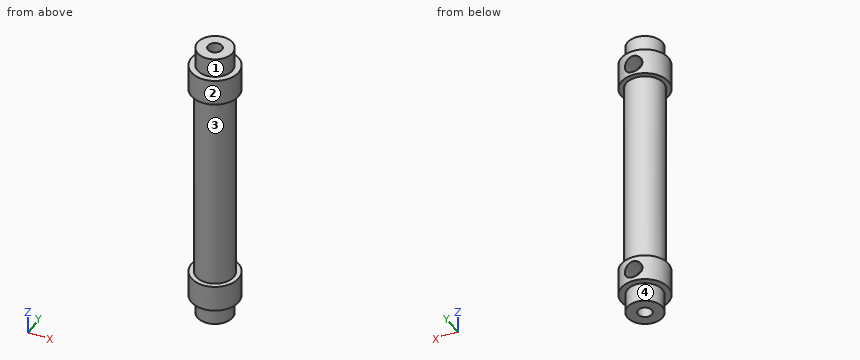
from build123d import *

# Parameters (mm, degrees)
SKETCH_1_R          = 10.75
SKETCH_1_R_2        = 9
EXTRUDE_1_DEPTH     = 115
SKETCH_2_R          = 13.5
EXTRUDE_2_DEPTH     = 15
SKETCH_3_R          = 10
EXTRUDE_3_DEPTH     = 11
SKETCH_4_R          = 4
CUT_EXTRUDE_4_DEPTH = 143.286682441
SKETCH_5_R          = 5
CUT_EXTRUDE_5_DEPTH = 15


with BuildPart() as part:
    # 草图1 → 拉伸1 (new body)
    with BuildSketch(Plane.XY):
        Circle(SKETCH_1_R)
        Circle(SKETCH_1_R_2, mode=Mode.SUBTRACT)
    extrude(amount=EXTRUDE_1_DEPTH)

    # 草图2 → 拉伸2 (add)
    with BuildSketch(Plane.XY.offset(115)):
        Circle(SKETCH_2_R)
    extrude_2 = extrude(amount=EXTRUDE_2_DEPTH)

    # 草图3 → 拉伸3 (add)
    with BuildSketch(Plane.XY.offset(130)):
        Circle(SKETCH_3_R)
    extrude_3 = extrude(amount=EXTRUDE_3_DEPTH)

    # 草图4 → 拉伸4 (cut, through all)
    with BuildSketch(Plane.XY.offset(141)):
        Circle(SKETCH_4_R)
    cut_extrude_4 = extrude(amount=-CUT_EXTRUDE_4_DEPTH, mode=Mode.SUBTRACT)

    # 镜向2: 拉伸2, 拉伸3, 拉伸4 across plane
    add(extrude_2.mirror(Plane(origin=(0, 0, 57.5), x_dir=(1, 0, 0), z_dir=(0, 0, -1))))
    add(extrude_3.mirror(Plane(origin=(0, 0, 57.5), x_dir=(1, 0, 0), z_dir=(0, 0, -1))))
    add(cut_extrude_4.mirror(Plane(origin=(0, 0, 57.5), x_dir=(1, 0, 0), z_dir=(0, 0, -1))), mode=Mode.SUBTRACT)

    # 草图5 → 拉伸5 (cut)
    with BuildSketch(Plane(origin=(0, 13.5, 0), x_dir=(-1, 0, 0), z_dir=(0, 1, 0))):
        with Locations(Location((0, 121.892959872, 0), (0, 0, 90))):
            Circle(SKETCH_5_R)
        with Locations(Location((0, -7.708924082, 0), (0, 0, 90))):
            Circle(SKETCH_5_R)
    extrude(amount=-CUT_EXTRUDE_5_DEPTH, mode=Mode.SUBTRACT)


solid = part.part
Geometry: final body of the model. Coordinates: model frame, mm. Face numbers are marked on the shaded views. A direction names the side the tool comes from. Give positions to 0.01 mm unless a question says otherwise; leave off trailing zeros. Order: outer loops, then holes, each group sorted by start corner. A loop starts at its lowest first (then second) coordinate and runs counter-clockwise, first axis right, second up. Notation, with made-up numbers: (-10, -8) -> (22, -8) arc R25 cw to (22, 28) -> close; hole circle Ø1 at (9, 81.25). An arc over 180 degrees is marked (long way). Write each question's results on one line, items separated by ' | '.
1) Line query: line 1 along Z through (x, y) = (6, 11); line 2 along Z through (x, y) = (4, -0.75); line 3 along Y through (x, z) = (0, -13.25). Output: solid intervals per line, ascending.
Geometry says:
line 1: z = -15 to 0, 115 to 130 | line 2: z = -26 to -10.71, -4.71 to 0, 115 to 118.89, 124.89 to 141 | line 3: y = -13.5 to -4, 4 to 13.5
2) Cut plane B-B (x = 0). Give the number of separate pieces and of enclosed holes in the cut face, and give its area (3 significant figures).
Geometry says:
separate pieces: 4 | enclosed holes: 0 | area: 1,050 mm²
3) Cut plane C-C (y = -6.5). Output: boundary loops of the cut face in (x, z).
Geometry says:
outline: (-11.83, -15) -> (-7.6, -15) -> (-7.6, -26) -> (7.6, -26) -> (7.6, -15) -> (11.83, -15) -> (11.83, 0) -> (8.56, 0) -> (8.56, 115) -> (11.83, 115) -> (11.83, 130) -> (7.6, 130) -> (7.6, 141) -> (-7.6, 141) -> (-7.6, 130) -> (-11.83, 130) -> (-11.83, 115) -> (-8.56, 115) -> (-8.56, 0) -> (-11.83, 0) -> close; hole (-6.22, 0) -> (6.22, 0) -> (6.22, 115) -> (-6.22, 115) -> close
4) Draft query along Z for the marked faces 3 and 4. Return one class per face: released by +Z, released by -Z, zero draft, split by the parting line, or undercut.
Geometry says:
face 3: undercut | face 4: zero draft
5) Cut plane A-A (z = 104). Output: boundary loops of the cut face in (x, y).
Geometry says:
outline: circle Ø21.5 at (0, 0); hole circle Ø18 at (0, 0)
6) First-contact query: pin 1 Ø6 at (x, z) = (-9, 54) entering from -Y; pin 2 Ø0.6 at (x, z) = (4.5, -7) entering from +Y; pin 3 Ø1.4 at (x, z) = (4.5, 121) entering from +Y. Flat tips, straight axial feed; report the tip coordinate or a pass-through.
Geometry says:
pin 1: stops at y = -8.92 | pin 2: stops at y = -1.5 | pin 3: stops at y = 12.63
7) Set-up query: the marked faces 1 and 2. Return all of +Z, -Z, +X, -X, +Y, -Y with unobstructed straight access to the full face (end or side cutting, diameter ignored); none if empty.
Geometry says:
face 1: +Z | face 2: +Z, -Z
